Part model, mm, in its own coordinate system. Round coordinates to 2 decimals unless told otherwise and drop trailing zeros. Loops run counter-clockwise (first coordinate to the right, second up) from the corner with the lowest first, then second, coordinate; pieces in that order, holes last.
(1) Probe probe 1 along X at (y, z) = (-139, -0.75); probe 2 along Y at (x, z) = (154, 1.2); probe 3 along Y at (x, z) = (283, 1.6). List the from-to ranges inside material, lowest first.
(2) Cut at A-A on y = -179.5. List the corners of the cut face in (x, z), then the cut area to 3 significant figures.
(3) Cut at B-B on z = 0.3. List the corners of the cut face in (x, y), then the cut area to 3 significant figures.
from build123d import *

# Parameters (mm, degrees)
F0_W     = 933
F0_H     = 567
F1_DEPTH = 2.5
F2_W     = 131
F2_H     = 131
F3_DEPTH = 5.001
F4_W     = 131
F4_H     = 131
F5_DEPTH = 5.001
F6_SIZE  = 1


with BuildPart() as f1:
    # F0 (on Top) → F1 (new body, symmetric)
    with BuildSketch(Plane.XY):
        Rectangle(F0_W, F0_H)
    extrude(amount=F1_DEPTH, both=True)

    # F2 (on face) → F3 (cut, through all)
    with BuildSketch(Plane.XY.offset(2.5)):
        with Locations((-263, -174)):
            Rectangle(F2_W, F2_H)
    extrude(amount=-F3_DEPTH, mode=Mode.SUBTRACT)

    # F4 (on face) → F5 (cut, through all)
    with BuildSketch(Plane.XY.offset(2.5)):
        with Locations((173, -174)):
            Rectangle(F4_W, F4_H)
    extrude(amount=-F5_DEPTH, mode=Mode.SUBTRACT)

    # F6
    f6_edges = [f1.edges().sort_by_distance(p)[0] for p in [
        (-466.5, 0, 2.5),
        (-466.5, 0, -2.5),
        (0, -283.5, -2.5),
        (0, -283.5, 2.5),
        (466.5, 0, -2.5),
        (466.5, 0, 2.5),
        (0, 283.5, 2.5),
        (0, 283.5, -2.5),
    ]]
    chamfer(f6_edges, length=F6_SIZE)


solid = f1.part
Final values:
1. probe 1: x = -466.5 to -328.5, -197.5 to 107.5, 238.5 to 466.5
1. probe 2: y = -283.5 to -239.5, -108.5 to 283.5
1. probe 3: y = -283.4 to 283.4
2. outline: (-466.5, -1.5) - (-465.5, -2.5) - (-328.5, -2.5) - (-328.5, 2.5) - (-465.5, 2.5) - (-466.5, 1.5) - close; (-197.5, -2.5) - (107.5, -2.5) - (107.5, 2.5) - (-197.5, 2.5) - close; (238.5, -2.5) - (465.5, -2.5) - (466.5, -1.5) - (466.5, 1.5) - (465.5, 2.5) - (238.5, 2.5) - close
2. area: 3,350 mm2
3. outline: (-466.5, -283.5) - (466.5, -283.5) - (466.5, 283.5) - (-466.5, 283.5) - close; hole (-328.5, -239.5) - (-197.5, -239.5) - (-197.5, -108.5) - (-328.5, -108.5) - close; hole (107.5, -239.5) - (238.5, -239.5) - (238.5, -108.5) - (107.5, -108.5) - close
3. area: 495,000 mm2
